For this review, take the finished solid that the model builds, in its own axes (mm). Face numbers are marked on the shaded views. A direction names the side the tool comes from. Coordinates: 2 decimals unless noted, no trailing zeros. Loops run counter-clockwise (first coordinate to the right, second up) from the corner with the lowest first, then second, coordinate; pieces in that order, holes last. Notation, with made-up numbers: M 60.5,28 L 71.5,28 A15 cw 71.5,32 Z; hole C 82,-18.5 d9. An arc over 180 degrees is marked long. Use one line per item in the form item = value.
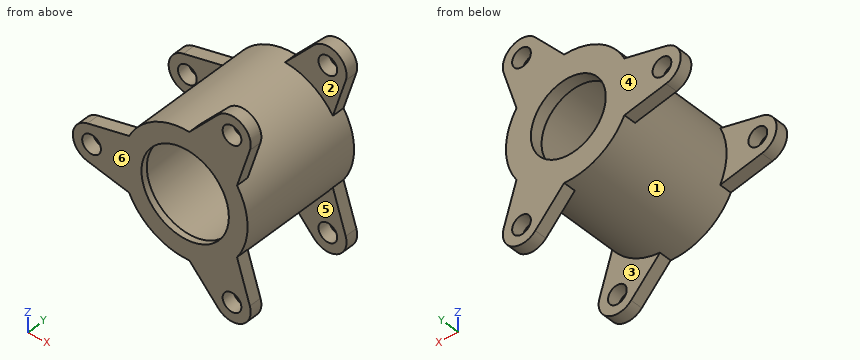
```python
from build123d import *

# Parameters (mm, degrees)
SKETCH2_R               = 7.5
BOSS_EXTRUDE1_DEPTH     = 10
CIRPATTERN1_COUNT       = 3
MIRROR1_COPY_1_SKETCH_R = 7.5
MIRROR1_COPY_1_DEPTH    = 10
MIRROR1_COPY_2_SKETCH_R = 7.5
MIRROR1_COPY_2_DEPTH    = 10


with BuildPart() as part:
    # Sketch1 → Revolve1 (revolve)
    with BuildSketch(Plane.XY):
        Polygon((35, 0), (35, 5), (40, 5), (40, 90), (30, 90), (30, 100), (50, 100), (50, 0), align=None)
    revolve(axis=Axis((0, 0, 0), (0, 1, 0)))

    # Sketch2 → Boss-Extrude1 (add)
    with BuildSketch(Plane(origin=(0, 100, 0), x_dir=(1, 0, 0), z_dir=(0, 1, 0))):
        with BuildLine():
            Line((-78.246594209, 14.644440107), (-44.879398453, 22.041769313))
            ThreePointArc((-44.879398453, 22.041769313), (-50, 0), (-44.879398453, -22.041769313))
            Line((-44.879398453, -22.041769313), (-78.246594209, -14.644440107))
            ThreePointArc((-78.246594209, -14.644440107), (-90, 0), (-78.246594209, 14.644440107))
        make_face()
        with Locations((-75, 0)):
            Circle(SKETCH2_R, mode=Mode.SUBTRACT)
    boss_extrude1 = extrude(amount=-BOSS_EXTRUDE1_DEPTH)

    # CirPattern1: Boss-Extrude1 ×3 about axis
    cirpattern1_axis = Axis((0, 0, 0), (0, 1, 0))
    for i in range(1, CIRPATTERN1_COUNT):
        add(boss_extrude1.rotate(cirpattern1_axis, i * 360 / CIRPATTERN1_COUNT))

    # Mirror1: Boss-Extrude1 across plane
    add(boss_extrude1.mirror(Plane.ZX.offset(50)))

    # Mirror1 copy 1 sketch → Mirror1 copy 1 (add)
    with BuildSketch(Plane(origin=(0, 0, 0), x_dir=(-0.5, 0, -0.866025404), z_dir=(0, -1, 0))):
        with BuildLine():
            Line((-78.246594209, -14.644440107), (-44.879398453, -22.041769313))
            ThreePointArc((-44.879398453, -22.041769313), (-50, 0), (-44.879398453, 22.041769313))
            Line((-44.879398453, 22.041769313), (-78.246594209, 14.644440107))
            ThreePointArc((-78.246594209, 14.644440107), (-90, 0), (-78.246594209, -14.644440107))
        make_face()
        with Locations((-75, 0)):
            Circle(MIRROR1_COPY_1_SKETCH_R, mode=Mode.SUBTRACT)
    extrude(amount=-MIRROR1_COPY_1_DEPTH)

    # Mirror1 copy 2 sketch → Mirror1 copy 2 (add)
    with BuildSketch(Plane(origin=(0, 0, 0), x_dir=(-0.5, 0, 0.866025404), z_dir=(0, -1, 0))):
        with BuildLine():
            Line((-78.246594209, -14.644440107), (-44.879398453, -22.041769313))
            ThreePointArc((-44.879398453, -22.041769313), (-50, 0), (-44.879398453, 22.041769313))
            Line((-44.879398453, 22.041769313), (-78.246594209, 14.644440107))
            ThreePointArc((-78.246594209, 14.644440107), (-90, 0), (-78.246594209, -14.644440107))
        make_face()
        with Locations((-75, 0)):
            Circle(MIRROR1_COPY_2_SKETCH_R, mode=Mode.SUBTRACT)
    extrude(amount=-MIRROR1_COPY_2_DEPTH)


solid = part.part
```
1. Consider section D-D on z = 52. Write out the cut boundary in (x, y), plus the area to 3 significant figures.
Computed values:
outline = M 5.29,0 L 49.14,0 L 49.14,10 L 5.29,10 Z; M 5.29,90 L 49.14,90 L 49.14,100 L 5.29,100 Z
area = 877 mm2
2. Wall thickness on line 1 along Z through (x, y) = (37.5, 93.5); line 2 along X through (y, z) = (2, 0); line 3 along X through (y, z) = (8.25, 0): over which ranges is each line inside the solid? List them lowest first. Write a range as from..to.
Computed values:
line_1 = -79.95..-72.45, -57.45..57.45, 72.45..79.95
line_2 = -90..-82.5, -67.5..-35, 35..50
line_3 = -90..-82.5, -67.5..-40, 40..50
3. Consider section A-A on x = 37. State how many separate pieces and enclosed holes the cut face has, plus the area to 3 significant figures.
Computed values:
separate_pieces = 5
enclosed_holes = 1
area = 5,400 mm2
4. Consider section C-C on x = 0. Write out the cut boundary in (y, z), plus the area to 3 significant figures.
Computed values:
outline = M 0,-50 L 100,-50 L 100,-30 L 90,-30 L 90,-40 L 5,-40 L 5,-35 L 0,-35 Z; M 0,35 L 5,35 L 5,40 L 90,40 L 90,30 L 100,30 L 100,50 L 0,50 Z
area = 2,250 mm2
5. Draft analysis for pull direction Y (two halves, no side actions). For the marked faces 4, 5 and 6, state which applies: +Y half, -Y half, draft (parallel to the pull), parting line (faces both ways), or undercut.
Computed values:
face_4 = +Y half
face_5 = undercut
face_6 = -Y half
6. Consider section B-B on z = 0. Write out the cut boundary in (x, y).
Computed values:
outline = M -90,0 L -82.5,0 L -82.5,10 L -90,10 Z; M -90,90 L -82.5,90 L -82.5,100 L -90,100 Z; M -67.5,0 L -35,0 L -35,5 L -40,5 L -40,90 L -30,90 L -30,100 L -67.5,100 L -67.5,90 L -50,90 L -50,10 L -67.5,10 Z; M 30,90 L 40,90 L 40,5 L 35,5 L 35,0 L 50,0 L 50,100 L 30,100 Z
7. Tool access review of the marked faces 1, 2 and 3: name each direction out of +Z, -Z, +X, -X, +Y, -Y from which nothing blocks a thin tool from reaching the whole face with its end or side.
Computed values:
face_1 = none
face_2 = +Z, +X
face_3 = -Z, +X
8. For pin 1 Ø10 at (y, z) = (20.5, -26) entering from -X; pin 2 Ø9 at (x, z) = (37.5, -64.95) entering from -Y; pin 3 Ø4 at (x, y) = (31, 75) entering from +Z; pin 4 Ø5 at (y, z) = (27, -29) entering from +X, all flat-tipped, find the tip position at first contact; note any pin that passes through.
Computed values:
pin_1 = -45.38
pin_2 = through
pin_3 = 40.73
pin_4 = 42.4
